The model under review builds one solid part; all positions refer to its coordinate system, in mm. A direction names the side the tool comes from. Round coordinates to 2 decimals unless told otherwise and drop trailing zeros. Write each loop counter-clockwise with the first axis right and the second up, starting at its lowest first coordinate (ties: lowest second). Pieces come first, ordered by that corner, then holes. Notation, with made-up numbers: (-28.5, 40) - (-21.5, 40) arc R17 cw to (-21.5, 52) - close; hole circle Ø1 at (72.5, -25). An arc over 180 degrees is marked (long way). Return JSON: item names as keys, results as strings.
Autodesk Inventor part; units mm, degrees
ref_plane "YZ Plane" through (0, 0, 0) normal (1, 0, 0) x (0, 1, 0)
ref_plane "XZ Plane" through (0, 0, 0) normal (0, 1, 0) x (-1, 0, 0)
ref_plane "XY Plane" through (0, 0, 0) normal (0, 0, 1) x (1, 0, 0)
sketch "Sketch1" plane through (0, 0, 0) normal (0, 0, 1) x (1, 0, 0)
  line L0 (0, 0) -> (0, 17.78)
  line L1 (0, 17.78) -> (25.4, 17.78)
  line L2 (25.4, 17.78) -> (25.4, 0)
  line L3 (25.4, 0) -> (0, 0)
  line L4 (0, 4) -> (25.4, 4)
  dimension "d0" = 17.78
  dimension "d1" = 25.4
  dimension "d2" = 4
revolve "Revolution1" add sketch "Sketch1" angle 360 about axis through (25.4, 0, 0) along (-1, 0, 0) contours L0 L1 L2 L4
sketch "Sketch2" plane through (25.4, 0, 0) normal (1, 0, 0) x (0, 0, -1)
  line L0 (-1.5875, 5.5875) -> (1.5875, 5.5875)
  line L1 (1.5875, 5.5875) -> (1.5875, 2.4125)
  line L2 (1.5875, 2.4125) -> (-1.5875, 2.4125)
  line L3 (-1.5875, 2.4125) -> (-1.5875, 5.5875)
  circle A0 centre (0, 0) radius 4
  line L4 (-1.5875, 5.5875) -> (1.5875, 2.4125) construction
  line L5 (1.5875, 5.5875) -> (-1.5875, 2.4125) construction
  point P0 (0, 4)
  dimension "d4" = 3.175
  dimension "d5" = 3.175
extrude "Extrusion1" cut sketch "Sketch2" against normal through all contours L0 L1 A0 L3 | A0 L1 L2 L3 picked at (0, 2.9417)
properties part number "SpacerB"
(1) Mouldability with a two-part tool opening along Y and no side actions: class faces 3 (the flat face through (25.4, -0.2, -4.2)), 4 (the flat face through (13, 5, -1.588)), 5 (the cylindrical face through (12.88, -3.85, -17.36)), 6 (the flat face through (13, 5, 1.588)) as released by +Y, released by -Y, zero draft, split by the parting line, or undercut.
Filled in:
{"face 3": "zero draft", "face 4": "undercut", "face 5": "split by the parting line", "face 6": "undercut"}
(2) Add section B-B (y = 5). Write out the cut boundary in (x, z).
Filled in:
{"outline": "(0, -17.06) - (25.4, -17.06) - (25.4, -1.59) - (0, -1.59) - close; (0, 1.59) - (25.4, 1.59) - (25.4, 17.06) - (0, 17.06) - close"}
(3) Add section D-D (z = 15). Write out the cut boundary in (x, y).
Filled in:
{"outline": "(0, -9.55) - (25.4, -9.55) - (25.4, 9.55) - (0, 9.55) - close"}
(4) Add section A-A (z = 0). Write out the cut boundary in (x, y).
Filled in:
{"outline": "(0, -17.78) - (25.4, -17.78) - (25.4, -4) - (0, -4) - close; (0, 5.59) - (25.4, 5.59) - (25.4, 17.78) - (0, 17.78) - close"}
(5) Add section C-C (x = 9.5). Write out the cut boundary in (y, z).
Filled in:
{"outline": "circle Ø35.56 at (0, 0); hole (3.67, -1.59) - (5.59, -1.59) - (5.59, 1.59) - (3.67, 1.59) arc R4 ccw (long way) to start"}
(6) For faces 1 (the flat face through (0, -0.2, -4.2)), 2 (the flat face through (13, 5.588, 0)), list the 3-axis set-ups (+Z, -Z, +X, -X, +Y, -Y) from which the entire face can be reached by the end or side of a thin tool; tool diameter is ignored.
Filled in:
{"face 1": "+Z, -Z, -X, +Y, -Y", "face 2": "+X, -X"}
(7) Clearance check with flat-ended pins moving along their axes: pin 1 Ø1.5 at (x, y) = (5, 8) entering from -Z; pin 2 Ø0.6 at (x, y) = (12, 4.5) entering from +Z; pin 3 Ø10 at (x, z) = (16, -6) entering from +Y; pin 4 Ø3.5 at (x, z) = (11.5, 0.5) entering from -Y. State where each tip first meets the part, or that it passes through.
Filled in:
{"pin 1": "stops at z = -16.23", "pin 2": "stops at z = 17.28", "pin 3": "stops at y = 17.75", "pin 4": "stops at y = -17.78"}
(8) Wall thickness on line 1 (Z direction, x = 13.25, y = 0); line 2 (Y direction, x = 14, z = 0); line 3 (Y direction, x = 17.5, z = 2.5): over which ranges is each line inside the solid? List them lowest first.
Filled in:
{"line 1": "z = -17.78 to -4, 4 to 17.78", "line 2": "y = -17.78 to -4, 5.59 to 17.78", "line 3": "y = -17.6 to -3.12, 3.12 to 17.6"}
